Verification items for the finished model (mm, model axes). A direction names the side the tool comes from. Give positions to 0.01 mm unless a question says otherwise; leave off trailing zeros. Order: outer loops, then holes, each group sorted by start corner. A loop starts at its lowest first (then second) coordinate and runs counter-clockwise, first axis right, second up.
from build123d import *

# Parameters (mm, degrees)
BOSS_EXTRUDE1_DEPTH      = 3
BOSS_EXTRUDE1_DEPTH_BACK = 6
SKETCH1_R                = 10
SKETCH4_R                = 1.6
HOLE_DEPTH               = 19.539009706
HOLECIR_COUNT            = 5
FILLET3_R                = 0.9
SKETCH5_R                = 3.5
CUT_EXTRUDE1_DEPTH       = 2.6
SKETCH6_R                = 1.6
CUT_EXTRUDE2_DEPTH       = 17.76305479


with BuildPart() as part:
    # Sketch1 → Boss-Extrude1 (new, two sides: drawn at the far end of the back side and taken through both)
    with BuildSketch(Plane(origin=(0, 0, 0), x_dir=(1, 0, 0), z_dir=(0, 1, 0)).offset(-BOSS_EXTRUDE1_DEPTH_BACK)):
        with Locations(Location((0, 0, 0), (0, 0, 270))):
            Circle(SKETCH1_R)
    extrude(amount=BOSS_EXTRUDE1_DEPTH + BOSS_EXTRUDE1_DEPTH_BACK)

    # Sketch4 → hole (cut, through all)
    with BuildSketch(Plane(origin=(-3.352872105, -1.093066116, 1.887711608), x_dir=(-0.4486862613641547, -0.14627571033740308, -0.8816371449912632), z_dir=(0.8382180262940947, 0.2732665289126682, -0.47192790187872385))):
        with Locations(Location((0, 0, 0), (0, 0, 8.746528197))):
            Circle(SKETCH4_R)
    hole = extrude(amount=-HOLE_DEPTH, mode=Mode.SUBTRACT)

    # holecir: hole ×5 about axis
    holecir_axis = Axis((0, 0, 0), (0, 1, 0))
    for i in range(1, HOLECIR_COUNT):
        add(hole.rotate(holecir_axis, i * 360 / HOLECIR_COUNT), mode=Mode.SUBTRACT)

    # Fillet3
    fillet3_edges = [part.edges().sort_by_distance(p)[0] for p in [
        (0, 3, -10),
    ]]
    fillet(fillet3_edges, radius=FILLET3_R)

    # Sketch5 → Cut-Extrude1 (cut)
    with BuildSketch(Plane.XZ.offset(6)):
        with Locations(Location((0, 0, 0), (0, 0, 270))):
            Circle(SKETCH5_R)
    extrude(amount=-CUT_EXTRUDE1_DEPTH, mode=Mode.SUBTRACT)

    # Sketch6 → Cut-Extrude2 (cut, through all)
    with BuildSketch(Plane(origin=(0, 3, 0), x_dir=(1, 0, 0), z_dir=(0, 1, 0))):
        with Locations(Location((-1.479875163, 7.352548504, 0), (0, 0, 270))):
            Circle(SKETCH6_R)
        with Locations(Location((5.518963734, -5.078487896, 0), (0, 0, 270))):
            Circle(SKETCH6_R)
    extrude(amount=-CUT_EXTRUDE2_DEPTH, mode=Mode.SUBTRACT)


solid = part.part
(1) Go/stop test with flat-tipped pins: pin 1 (4 mm diameter, centred on x = 0, z = 0, fed in from -Y); pin 2 (5 mm diameter, centred on x = -5, y = -3, fed in from +Z); pin 3 (3 mm diameter, centred on y = -2.5, z = 1.5, fed in from +X). Record where each tip stops, or that it passes through.
Solved:
pin 1: stops at y = -3.4
pin 2: stops at z = 9.68
pin 3: stops at x = 9.98
(2) Section check C-C, the plane y = 1.5. Enter the section's corners in (x, z).
Solved:
outline: circle Ø20 at (0, 0); hole circle Ø3.2 at (-1.48, -7.35); hole circle Ø3.2 at (5.52, 5.08)
(3) Scan lines: line 1 (X direction, y = -0.5, z = 5.5); line 2 (X direction, y = -3.5, z = -7); line 3 (Z direction, x = -1, y = -3.5). Record each from-to range of solid material in increasing order.
Solved:
line 1: x = -8.35 to -0.18, 2.28 to 3.98, 7.06 to 8.35
line 2: x = -5.68 to -3.04, 0.08 to 2.29, 4.47 to 7.14
line 3: z = -9.95 to -8.88, -5.83 to -3.35, 3.35 to 9.95
(4) Set-up check for faces 1 (the flat face through (0, 3, 0)), 2 (the flat face through (0.782, -1.072, 3.774)), 3 (the cylindrical face through (-3.417, -4.718, 0.759)): record each of +Z, -Z, +X, -X, +Y, -Y from which the full face is reachable in a straight line by a thin tool's end or side.
Solved:
face 1: +Z, -Z, +X, -X, +Y
face 2: none
face 3: -Y
(5) Section check A-A, the plane x = 6.25. Give the number of separate pieces and of enclosed holes in the cut face, then the cut area to 3 significant figures.
Solved:
separate pieces: 2
enclosed holes: 1
area: 106 mm2
(6) Release check for a two-part mould opening along Z. For faces 4 (the cylindrical face through (-5.14, -3.52, -4.26)), 5 (the cylindrical face through (2.463, -3.518, -6.208)), 6 (the cylindrical face through (0, -2, -10)), 7 (the flat face through (-4, -6, 0)) record: pulls with the +Z half, pulls with the -Z half, needs draft (parallel to the pull), parting line crosses it, or undercut.
Solved:
face 4: undercut
face 5: undercut
face 6: parting line crosses it
face 7: needs draft
